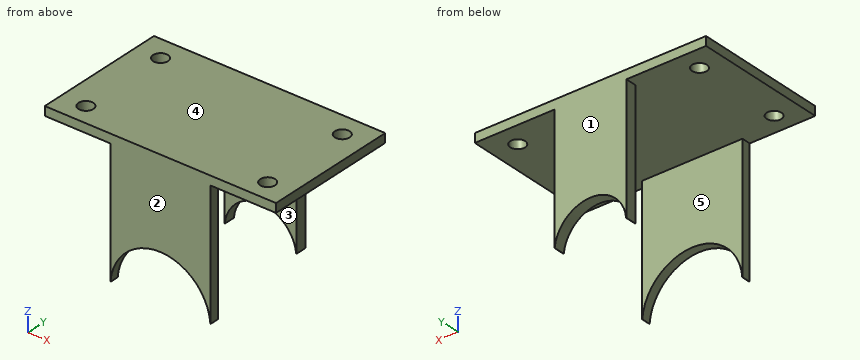
from build123d import *

# Parameters (mm, degrees)
SKETCH1_W           = 51.4
SKETCH1_H           = 30
BOSS_EXTRUDE1_DEPTH = 2
SKETCH2_R           = 1.65
CUT_EXTRUDE1_DEPTH  = 15
SKETCH3_W           = 16
SKETCH3_H           = 2.5
SKETCH3_W_2         = 22.3
SKETCH3_H_2         = 2
BOSS_EXTRUDE2_DEPTH = 28
SKETCH4_R           = 8
CUT_EXTRUDE3_DEPTH  = 10
SKETCH6_R           = 11.15
CUT_EXTRUDE4_DEPTH  = 10


with BuildPart() as part:
    # Sketch1 → Boss-Extrude1 (new body)
    with BuildSketch(Plane.XY):
        with Locations((25.7, 15)):
            Rectangle(SKETCH1_W, SKETCH1_H)
    extrude(amount=BOSS_EXTRUDE1_DEPTH)

    # Sketch2 → Cut-Extrude1 (cut)
    with BuildSketch(Plane(origin=(0, 0, 0), x_dir=(-1, 0, 0), z_dir=(0, 0, -1))):
        with Locations((-45.9, 25)):
            Circle(SKETCH2_R)
        with Locations((-5.5, 25)):
            Circle(SKETCH2_R)
        with Locations((-5.5, 4.5)):
            Circle(SKETCH2_R)
        with Locations((-45.9, 4.5)):
            Circle(SKETCH2_R)
    extrude(amount=-CUT_EXTRUDE1_DEPTH, mode=Mode.SUBTRACT)

    # Sketch3 → Boss-Extrude2 (add)
    with BuildSketch(Plane(origin=(0, 0, 0), x_dir=(-1, 0, 0), z_dir=(0, 0, -1))):
        with Locations((-25.7, 28.75)):
            Rectangle(SKETCH3_W, SKETCH3_H)
        with Locations((-25.7, 1)):
            Rectangle(SKETCH3_W_2, SKETCH3_H_2)
    extrude(amount=BOSS_EXTRUDE2_DEPTH)

    # Sketch4 → Cut-Extrude3 (cut)
    with BuildSketch(Plane(origin=(0, 30, 0), x_dir=(1, 0, 0), z_dir=(0, 1, 0))):
        with Locations((25.7, 28.85)):
            Circle(SKETCH4_R)
    extrude(amount=-CUT_EXTRUDE3_DEPTH, mode=Mode.SUBTRACT)

    # Sketch6 → Cut-Extrude4 (cut)
    with BuildSketch(Plane(origin=(0, 2, 0), x_dir=(1, 0, 0), z_dir=(0, 1, 0))):
        with Locations((25.7, 28.85)):
            Circle(SKETCH6_R)
    extrude(amount=-CUT_EXTRUDE4_DEPTH, mode=Mode.SUBTRACT)


solid = part.part
Here's how the part is built. I have some questions about the finished solid (model axes, mm). Face numbers are marked on the shaded views. A direction names the side the tool comes from. Coordinates: 2 decimals unless noted, no trailing zeros. Write each loop counter-clockwise with the first axis right and the second up, starting at its lowest first coordinate (ties: lowest second). Pieces come first, ordered by that corner, then holes.
Item 1: If we mould it in two halves opening along Y, with no side actions, what happens to the marked faces 1, 2 and 3? For each: +Y half, -Y half, draft (parallel to the pull), parting line (faces both ways), or undercut.
Item 2: I want a section at B-B on y = 25. Write out the boundary of the cut face in (x, z).
Item 3: I want a section at C-C on x = 45.9. Write out the boundary of the cut face in (y, z), and give its area (3 significant figures).
Item 4: I want a section at D-D on z = -25. Write out the boundary of the cut face in (x, y), and give its area (3 significant figures).
Item 5: Will these pins go through, and if not, where does the flat tip stop? pin 1 (5.5 mm diameter, centred on x = 5.5, y = 4.5, fed in from -Z); pin 2 (3 mm diameter, centred on y = 29, z = -10.5, fed in from +X); pin 3 (1.2 mm diameter, centred on y = 29, z = -7.5, fed in from -X).
Item 6: I want a section at A-A on z = -5. Write out the boundary of the cut face in (x, y).
Item 7: On a 3-axis mill with a long thin cutter (end or side, diameter ignored), from which of +Z, -Z, +X, -X, +Y, -Y can I reach the whole of each face in a straight line? I mean the marked faces 4 and 5. Say none if no direction works.
Item 8: If I drill on line 1 (Y direction, x = 5.5, z = 1.6); line 2 (Y direction, x = 24.5, z = -17); line 3 (Z direction, x = 5.5, y = 14.75), over which ranges is the centre line in solid material (lowest first)?
Findings below:
1. face 1: +Y half
1. face 2: -Y half
1. face 3: undercut
2. outline: (0, 0) - (3.85, 0) - (3.85, 2) - (0, 2) - close; (7.15, 0) - (44.25, 0) - (44.25, 2) - (7.15, 2) - close; (47.55, 0) - (51.4, 0) - (51.4, 2) - (47.55, 2) - close
3. outline: (0, 0) - (2.85, 0) - (2.85, 2) - (0, 2) - close; (6.15, 0) - (23.35, 0) - (23.35, 2) - (6.15, 2) - close; (26.65, 0) - (30, 0) - (30, 2) - (26.65, 2) - close
3. area: 46.8 mm2
4. outline: (14.55, 0) - (15.24, 0) - (15.24, 2) - (14.55, 2) - close; (17.7, 27.5) - (18.69, 27.5) - (18.69, 30) - (17.7, 30) - close; (32.71, 27.5) - (33.7, 27.5) - (33.7, 30) - (32.71, 30) - close; (36.16, 0) - (36.85, 0) - (36.85, 2) - (36.16, 2) - close
4. area: 7.68 mm2
5. pin 1: stops at z = 0
5. pin 2: stops at x = 33.7
5. pin 3: stops at x = 17.7
6. outline: (14.55, 0) - (36.85, 0) - (36.85, 2) - (14.55, 2) - close; (17.7, 27.5) - (33.7, 27.5) - (33.7, 30) - (17.7, 30) - close
7. face 4: +Z, +X, -X, +Y, -Y
7. face 5: -Z, +X, -X
8. line 1: y = 0 to 2.85, 6.15 to 23.35, 26.65 to 30
8. line 2: y = 0 to 2, 27.5 to 30
8. line 3: z = 0 to 2
